from build123d import *

# Parameters (mm, degrees)
SKETCH_1_W          = 35
SKETCH_1_H          = 36
EXTRUDE_1_DEPTH     = 2
CUT_EXTRUDE_1_REACH = 27.184


with BuildPart() as part:
    # 草图1 → 凸台-拉伸1 (new body)
    with BuildSketch(Plane.XY):
        Rectangle(SKETCH_1_W, SKETCH_1_H)
    extrude(amount=EXTRUDE_1_DEPTH)

    # 草图2 → 切除-拉伸1 (cut, up to next)
    with BuildSketch(Plane.XY.offset(2), mode=Mode.PRIVATE) as cut_extrude_1_sk1:
        with BuildLine():
            Line((-7.5, 9), (7.5, 9))
            ThreePointArc((7.5, 9), (8.5, 8), (7.5, 7))
            Line((7.5, 7), (-7.5, 7))
            ThreePointArc((-7.5, 7), (-8.5, 8), (-7.5, 9))
        make_face()
    cut_extrude_1_tool1 = extrude(cut_extrude_1_sk1.sketch, amount=-CUT_EXTRUDE_1_REACH, mode=Mode.PRIVATE) & part.part
    # 草图2 → 切除-拉伸1 (cut, up to next)
    with BuildSketch(Plane.XY.offset(2), mode=Mode.PRIVATE) as cut_extrude_1_sk2:
        with BuildLine():
            Line((-7.509739979, 1), (7.490260021, 1))
            ThreePointArc((7.490260021, 1), (8.490260021, 0), (7.490260021, -1))
            Line((7.490260021, -1), (-7.509739979, -1))
            ThreePointArc((-7.509739979, -1), (-8.509739979, 0), (-7.509739979, 1))
        make_face()
    cut_extrude_1_tool2 = extrude(cut_extrude_1_sk2.sketch, amount=-CUT_EXTRUDE_1_REACH, mode=Mode.PRIVATE) & part.part
    # 草图2 → 切除-拉伸1 (cut, up to next)
    with BuildSketch(Plane.XY.offset(2), mode=Mode.PRIVATE) as cut_extrude_1_sk3:
        with BuildLine():
            Line((-7.285332316, -7), (7.714667684, -7))
            ThreePointArc((7.714667684, -7), (8.714667684, -8), (7.714667684, -9))
            Line((7.714667684, -9), (-7.285332316, -9))
            ThreePointArc((-7.285332316, -9), (-8.285332316, -8), (-7.285332316, -7))
        make_face()
    cut_extrude_1_tool3 = extrude(cut_extrude_1_sk3.sketch, amount=-CUT_EXTRUDE_1_REACH, mode=Mode.PRIVATE) & part.part
    add(cut_extrude_1_tool1.solids().sort_by_distance((0, 8, 2))[0], mode=Mode.SUBTRACT)
    add(cut_extrude_1_tool2.solids().sort_by_distance((-0.00974, 0, 2))[0], mode=Mode.SUBTRACT)
    add(cut_extrude_1_tool3.solids().sort_by_distance((0.214668, -8, 2))[0], mode=Mode.SUBTRACT)


solid = part.part
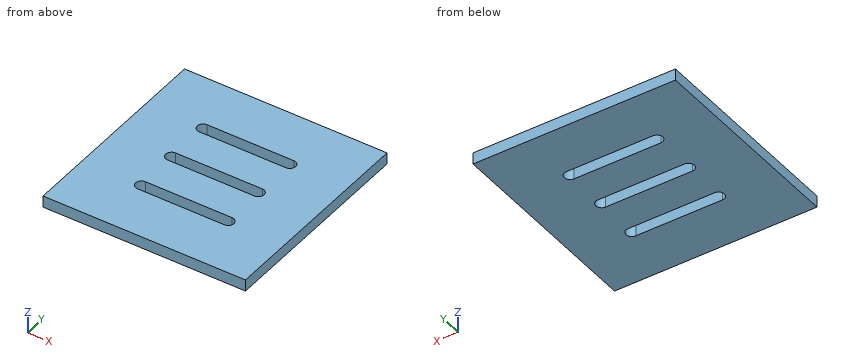
Input: part model. Units: mm. Frame: model coordinates. Give positions to 0.01 mm unless a question says otherwise; leave off trailing zeros. Order: outer loops, then holes, each group sorted by start corner. A loop starts at its lowest first (then second) coordinate and runs counter-clockwise, first axis right, second up.
Q1. Section A-A on x = 0.5. Output: boundary loops of the cut face in (y, z), and give its area (3 significant figures).
Checked values:
outline: (-18, 0) - (-9, 0) - (-9, 2) - (-18, 2) - close; (-7, 0) - (-1, 0) - (-1, 2) - (-7, 2) - close; (1, 0) - (7, 0) - (7, 2) - (1, 2) - close; (9, 0) - (18, 0) - (18, 2) - (9, 2) - close
area: 60.0 mm2
Q2. Section B-B on z = 1.2. Output: boundary loops of the cut face in (x, y).
Checked values:
outline: (-17.5, -18) - (17.5, -18) - (17.5, 18) - (-17.5, 18) - close; hole (-7.51, -1) - (7.49, -1) arc R1 ccw to (7.49, 1) - (-7.51, 1) arc R1 ccw to start; hole (-7.5, 7) - (7.5, 7) arc R1 ccw to (7.5, 9) - (-7.5, 9) arc R1 ccw to start; hole (-7.29, -9) - (7.71, -9) arc R1 ccw to (7.71, -7) - (-7.29, -7) arc R1 ccw to start
Q3. Section C-C on y = 0. Output: boundary loops of the cut face in (x, z).
Checked values:
outline: (-17.5, 0) - (-8.51, 0) - (-8.51, 2) - (-17.5, 2) - close; (8.49, 0) - (17.5, 0) - (17.5, 2) - (8.49, 2) - close
Q4. Ray query, probe 1 along Y at (x, z) = (-7, 1.6); probe 2 along X at (y, z) = (-8, 1.6); probe 3 along X at (y, z) = (-8.5, 0.7). Return the intervals inside material, ascending.
Checked values:
probe 1: y = -18 to -9, -7 to -1, 1 to 7, 9 to 18
probe 2: x = -17.5 to -8.29, 8.71 to 17.5
probe 3: x = -17.5 to -8.15, 8.58 to 17.5
